Design review of the part built by this model. Coordinates are the model's own, in mm. A direction names the side the tool comes from. Give positions to 0.01 mm unless a question says otherwise; leave off trailing zeros. Write each loop counter-clockwise with the first axis right and the second up, starting at its lowest first coordinate (ties: lowest second). Pieces come first, ordered by that corner, then holes. Notation, with made-up numbers: (24.25, -38) -> (57.25, -38) arc R25 ccw to (57.25, -5) -> close; hole circle Ø5 at (-5.75, 13). An arc over 180 degrees is marked (long way). Use CSV: the item, a comma, the result in double quotes.
```python
from build123d import *

# Parameters (mm, degrees)
BOSS_EXTRUDE1_DEPTH     = 17.5
CUT_EXTRUDE1_DEPTH      = 10
CUT_EXTRUDE1_DEPTH_BACK = 34.260336739
CUT_EXTRUDE1_START      = -20
SKETCH3_R               = 3.375
SKETCH3_R_2             = 1.875
CUT_EXTRUDE6_DEPTH      = 34.260336739
CUT_EXTRUDE6_DEPTH_BACK = 34.260336739
SKETCH3_4_R             = 1.875
SKETCH3_4_R_2           = 3


with BuildPart() as part:
    # Sketch1 → Boss-Extrude1 (new, symmetric)
    with BuildSketch(Plane(origin=(0, 0, 0), x_dir=(1, 0, 0), z_dir=(0, 1, 0))):
        Polygon((-20, 20), (20, 20), (20, -10), (10, -10), (10, 10), (-10, 10), (-10, -10), (-20, -10), align=None)
    extrude(amount=BOSS_EXTRUDE1_DEPTH, both=True)

    # Sketch3 → Cut-Extrude1 (cut, two sides: drawn at the far end of the back side and taken through both)
    # profile 1 of 4: a face of its own
    with BuildSketch(Plane.XY.offset(CUT_EXTRUDE1_START - CUT_EXTRUDE1_DEPTH_BACK)):
        with Locations((-14, 12.5)):
            Circle(SKETCH3_R)
        with Locations((-14, 12.5)):
            Circle(SKETCH3_R_2, mode=Mode.SUBTRACT)
    # profile 2 of 4: a face of its own
    with BuildSketch(Plane.XY.offset(CUT_EXTRUDE1_START - CUT_EXTRUDE1_DEPTH_BACK)):
        with Locations((14, 12.5)):
            Circle(SKETCH3_R)
        with Locations((14, 12.5)):
            Circle(SKETCH3_R_2, mode=Mode.SUBTRACT)
    # profile 3 of 4: a face of its own
    with BuildSketch(Plane.XY.offset(CUT_EXTRUDE1_START - CUT_EXTRUDE1_DEPTH_BACK)):
        with Locations((14, -12.5)):
            Circle(SKETCH3_R)
        with Locations((14, -12.5)):
            Circle(SKETCH3_R_2, mode=Mode.SUBTRACT)
    # profile 4 of 4: a face of its own
    with BuildSketch(Plane.XY.offset(CUT_EXTRUDE1_START - CUT_EXTRUDE1_DEPTH_BACK)):
        with Locations((-14, -12.5)):
            Circle(SKETCH3_R)
        with Locations((-14, -12.5)):
            Circle(SKETCH3_R_2, mode=Mode.SUBTRACT)
    extrude(amount=CUT_EXTRUDE1_DEPTH + CUT_EXTRUDE1_DEPTH_BACK, mode=Mode.SUBTRACT)

    # Sketch3<4> → Cut-Extrude6 (cut, two sides: drawn at the far end of the back side and taken through both)
    with BuildSketch(Plane.XY.offset(-CUT_EXTRUDE6_DEPTH_BACK)):
        with Locations((-14, 12.5)):
            Circle(SKETCH3_4_R)
        with Locations((-14, -12.5)):
            Circle(SKETCH3_4_R)
        with Locations((14, -12.5)):
            Circle(SKETCH3_4_R)
        with Locations((14, 12.5)):
            Circle(SKETCH3_4_R)
        Circle(SKETCH3_4_R_2)
    extrude(amount=CUT_EXTRUDE6_DEPTH + CUT_EXTRUDE6_DEPTH_BACK, mode=Mode.SUBTRACT)


solid = part.part
```
(1) Take a section at C-C (y = 12.5). Write out the cut boundary in (x, z) (3 decimals), then the cut area to 3 significant figures.
Established:
outline,"(-20, -20) -> (-17.375, -20) -> (-17.375, -10) -> (-15.875, -10) -> (-15.875, 10) -> (-20, 10) -> close; (-12.125, -10) -> (-10.625, -10) -> (-10.625, -20) -> (10.625, -20) -> (10.625, -10) -> (12.125, -10) -> (12.125, 10) -> (10, 10) -> (10, -10) -> (-10, -10) -> (-10, 10) -> (-12.125, 10) -> close; (15.875, -10) -> (17.375, -10) -> (17.375, -20) -> (20, -20) -> (20, 10) -> (15.875, 10) -> close"
area,"515 mm2"
(2) Mouldability with a two-part tool opening along X and no side actions: class faces 1 (the face through (0, 4, -10)), 2 (the face through (0, 4, -20)), 3 (the face through (20, 0, -5)) as +X half, -X half, draft (parallel to the pull), parting line (faces both ways), or undercut.
Established:
face 1,"undercut"
face 2,"draft"
face 3,"+X half"
(3) Clearance check with flat-ended pins moving along their axes: pin 1 (9.5 mm diameter, centred on x = 0, y = 0, fed in from +Z); pin 2 (6 mm diameter, centred on x = -14, y = -12.5, fed in from -Z). State where each tip first meets the part, or that it passes through.
Established:
pin 1,"stops at z = -10"
pin 2,"stops at z = -10"
(4) Take a section at B-B (x = -14). Write out the cut boundary in (y, z) (3 decimals), then the cut area to 3 significant figures.
Established:
outline,"(-17.5, -20) -> (-15.875, -20) -> (-15.875, -10) -> (-14.375, -10) -> (-14.375, 10) -> (-17.5, 10) -> close; (-10.625, -10) -> (-9.125, -10) -> (-9.125, -20) -> (9.125, -20) -> (9.125, -10) -> (10.625, -10) -> (10.625, 10) -> (-10.625, 10) -> close; (14.375, -10) -> (15.875, -10) -> (15.875, -20) -> (17.5, -20) -> (17.5, 10) -> (14.375, 10) -> close"
area,"765 mm2"
(5) Take a section at D-D (y = -2). Write out the cut boundary in (x, z).
Established:
outline,"(-20, -20) -> (-2.24, -20) -> (-2.24, -10) -> (-10, -10) -> (-10, 10) -> (-20, 10) -> close; (2.24, -20) -> (20, -20) -> (20, 10) -> (10, 10) -> (10, -10) -> (2.24, -10) -> close"
(6) Tool access review of faces 4 (the face through (15.5, -14, -10)), 5 (the face through (-14.41, 10.67, -0.14)), 6 (the face through (-10, 0, 0)): name each direction out of +Z, -Z, +X, -X, +Y, -Y from which nothing blocks a thin tool from reaching the whole face with its end or side.
Established:
face 4,"-Z"
face 5,"+Z, -Z"
face 6,"+Z, +Y, -Y"
(7) For line 1 along X through (y, z) = (12.5, -3.5) (3 decimals); line 2 along X through (y, z) = (-12.5, -16.25) (3 decimals); line 3 along X through (y, z) = (14.5, -1.25), list the stretches that pass through material, from the lowest coordinate up. Write a range as [from, to].
Established:
line 1,"x = [-20, -15.875], [-12.125, -10], [10, 12.125], [15.875, 20]"
line 2,"x = [-20, -17.375], [-10.625, 10.625], [17.375, 20]"
line 3,"x = [-20, -10], [10, 20]"
(8) Take a section at A-A (z = -9). Write out the cut boundary in (x, y) (3 decimals).
Established:
outline,"(-20, -17.5) -> (-10, -17.5) -> (-10, 17.5) -> (-20, 17.5) -> close; (10, -17.5) -> (20, -17.5) -> (20, 17.5) -> (10, 17.5) -> close; hole circle Ø3.75 at (-14, -12.5); hole circle Ø3.75 at (-14, 12.5); hole circle Ø3.75 at (14, -12.5); hole circle Ø3.75 at (14, 12.5)"
